Geometry check sheet. Reference: the model listing, model coordinates, mm. Face numbers are marked on the shaded views. A direction names the side the tool comes from. Round coordinates to 2 decimals unless told otherwise and drop trailing zeros. Order: outer loops, then holes, each group sorted by start corner. A loop starts at its lowest first (then second) coordinate and runs counter-clockwise, first axis right, second up. Notation, with made-up numbers: (-34.5, 65.25) - (-29.5, 65.25) arc R10 cw to (-29.5, 74.25) - close; hole circle Ø4 at (17.5, -1). An arc over 180 degrees is marked (long way). Write each question's results on one line, items separated by ' | '.
```python
from build123d import *

# Parameters (mm, degrees)
SKETCH1_R             = 4.765
BOSS_EXTRUDE1_DEPTH   = 9.5
CHAMFER1_SIZE         = 2.54
CHAMFER1_SIZE2        = 7.62
CHAMFER1_PART_2_SIZE  = 2.54
CHAMFER1_PART_2_SIZE2 = 7.62
CHAMFER2_SIZE         = 7.62
CHAMFER2_SIZE2        = 2.54
CUT_EXTRUDE1_DEPTH    = 17
SKETCH3_W             = 9.53
SKETCH3_H             = 9.53
CUT_EXTRUDE2_DEPTH    = 17
SKETCH4_R             = 1.59
CUT_EXTRUDE3_DEPTH    = 17


with BuildPart() as part:
    # Sketch1 → Boss-Extrude1 (new body, symmetric)
    with BuildSketch(Plane(origin=(0, 0, 0), x_dir=(0, 0, -1), z_dir=(1, 0, 0))):
        with BuildLine():
            Line((0, 9.765), (-22.53, 9.765))
            Line((-22.53, 9.765), (-22.53, 4.765))
            Line((-22.53, 4.765), (-9.688074689, -1.223288118))
            ThreePointArc((-9.688074689, -1.223288118), (-5.812387316, -7.84674319), (1.653013564, -9.624072483))
            Line((1.653013564, -9.624072483), (28.575, -5))
            Line((28.575, -5), (28.575, 0))
            Line((28.575, 0), (9.765, 0))
            ThreePointArc((9.765, 0), (6.904897718, 6.904897718), (0, 9.765))
        make_face()
        Circle(SKETCH1_R, mode=Mode.SUBTRACT)
    extrude(amount=BOSS_EXTRUDE1_DEPTH, both=True)

    # Chamfer1
    chamfer1_edges = [part.edges().sort_by_distance(p)[0] for p in [
        (9.5, 7.265, 22.53),
    ]]
    chamfer1_side = [part.faces().sort_by_distance(p)[0] for p in [
        (0, 7.265, 22.53),
    ]]
    chamfer(chamfer1_edges, length=CHAMFER1_SIZE, length2=CHAMFER1_SIZE2, reference=chamfer1_side[0])

    # Chamfer1 part 2
    chamfer1_part_2_edges = [part.edges().sort_by_distance(p)[0] for p in [
        (9.5, -2.5, -28.575),
    ]]
    chamfer1_part_2_side = [part.faces().sort_by_distance(p)[0] for p in [
        (0, -2.5, -28.575),
    ]]
    chamfer(chamfer1_part_2_edges, length=CHAMFER1_PART_2_SIZE, length2=CHAMFER1_PART_2_SIZE2, reference=chamfer1_part_2_side[0])

    # Chamfer2
    chamfer2_edges = [part.edges().sort_by_distance(p)[0] for p in [
        (-9.5, 7.265, 22.53),
        (-9.5, -2.5, -28.575),
    ]]
    chamfer2_side = [part.faces().sort_by_distance(p)[0] for p in [
        (-9.5, 9.217903854, 11.265),
    ]]
    chamfer(chamfer2_edges, length=CHAMFER2_SIZE, length2=CHAMFER2_SIZE2, reference=chamfer2_side[0])

    # Sketch2 → Cut-Extrude1 (cut, symmetric)
    with BuildSketch(Plane(origin=(0, 0, 0), x_dir=(1, 0, 0), z_dir=(0, 1, 0))):
        with BuildLine():
            Line((5.08, 6.35), (5.08, -3.81))
            ThreePointArc((5.08, -3.81), (0, -8.89), (-5.08, -3.81))
            Line((-5.08, -3.81), (-5.08, 6.35))
            ThreePointArc((-5.08, 6.35), (0, 11.43), (5.08, 6.35))
        make_face()
    extrude(amount=CUT_EXTRUDE1_DEPTH, both=True, mode=Mode.SUBTRACT)

    # Sketch3 → Cut-Extrude2 (cut, symmetric)
    with BuildSketch(Plane(origin=(0, 0, 0), x_dir=(1, 0, 0), z_dir=(0, 1, 0))):
        with Locations((0, 23.81)):
            Rectangle(SKETCH3_W, SKETCH3_H)
        with Locations((0, -17.765)):
            Rectangle(SKETCH3_W, SKETCH3_H)
    extrude(amount=CUT_EXTRUDE2_DEPTH, both=True, mode=Mode.SUBTRACT)

    # Sketch4 → Cut-Extrude3 (cut, symmetric)
    with BuildSketch(Plane(origin=(0, 0, 0), x_dir=(0, 0, -1), z_dir=(1, 0, 0))):
        with Locations((26.035, -2.54)):
            Circle(SKETCH4_R)
        with Locations((-19.99, 7.225)):
            Circle(SKETCH4_R)
    extrude(amount=CUT_EXTRUDE3_DEPTH, both=True, mode=Mode.SUBTRACT)


solid = part.part
```
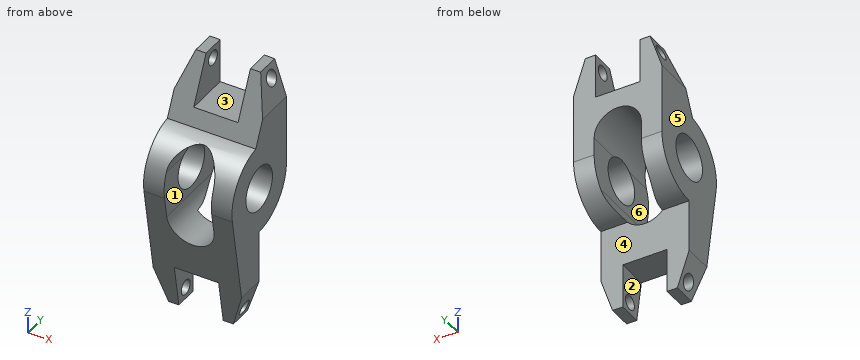
(1) Section check C-C (x = 0). Record the cut outline in (y, z) (3 decimals).
Answers follow:
outline: (-7.945, -11.43) - (-6.637, -19.045) - (0, -19.045) - (0, -11.43) - close; (-4.04, 8.89) - (9.765, 8.89) - (9.765, 13) - (0.321, 13) - (-1.223, 9.688) arc R9.765 ccw to start
(2) Access from +Z, -Z, +X, -X, +Y, -Y to the whole of each face (thin tool, end or side, straight path). Record for the marked faces 1, 2 and 3.
Answers follow:
face 1: +Y, -Y | face 2: -Z, +Y, -Y | face 3: +Z, +Y, -Y
(3) Draft check along X on the marked faces 4, 5 and 6. Enter one of: released by +X, released by -X, zero draft, split by the parting line, or undercut.
Answers follow:
face 4: zero draft | face 5: released by -X | face 6: undercut
(4) Section check A-A (y = 4). Record the cut outline in (x, z) (3 decimals), then the cut area to 3 significant figures.
Answers follow:
outline: (-9.5, -8.908) - (-4.389, -8.908) arc R5.08 cw to (-5.08, -6.35) - (-5.08, -2.589) - (-9.5, -2.589) - close; (-9.5, 2.589) - (-5.08, 2.589) - (-5.08, 3.81) arc R5.08 cw to (5.08, 3.81) - (5.08, 2.589) - (9.5, 2.589) - (9.5, 14.91) - (7.507, 20.889) - (4.765, 20.889) - (4.765, 13) - (-4.765, 13) - (-4.765, 20.889) - (-7.507, 20.889) - (-9.5, 14.91) - close; (4.389, -8.908) - (9.5, -8.908) - (9.5, -2.589) - (5.08, -2.589) - (5.08, -6.35) arc R5.08 cw to start | area: 265 mm²
(5) Material ranges on line 1 (X direction, y = -4.25, z = -5.5); line 2 (Y direction, x = -6.4, z = 19.99) (3 decimals); line 3 (Z direction, x = 4.5, y = -2.25) (3 decimals), recorded low to high.
Answers follow:
line 1: -9.5 to -5.08, 5.08 to 9.5 | line 2: 3.581 to 5.635, 8.815 to 9.765 | line 3: -19.045 to -8.707, 6.167 to 9.502
(6) Section check B-B (x = -6). Record the cut outline in (y, z) (3 decimals).
Answers follow:
outline: (-9.624, -1.653) - (-5, -28.575) - (0, -28.575) - (0, -9.765) arc R9.765 ccw to (9.765, 0) - (9.765, 22.53) - (4.765, 22.53) - (-1.223, 9.688) arc R9.765 ccw to start; hole circle Ø9.53 at (0, 0); hole circle Ø3.18 at (-2.54, -26.035); hole circle Ø3.18 at (7.225, 19.99)
(7) Depth check by flat-ended pin: pin 1 Ø5.5 at (x, y) = (-1, -2.5) entering from -Z (3 decimals); pin 2 Ø5 at (y, z) = (3.5, -12.5) entering from -X; pin 3 Ø5 at (y, z) = (-2.54, -26.035) entering from -X; pin 4 Ø4 at (y, z) = (7.225, 19.99) entering from +X. Enter the tip coordinate at first touch or a pass-through.
Answers follow:
pin 1: z = -19.045 | pin 2: through | pin 3: x = -8.64 | pin 4: x = 8.47
(8) Section check D-D (z = -16.5). Record the cut outline in (x, y), then the cut area to 3 significant figures.
Answers follow:
outline: (-9.5, -7.07) - (9.5, -7.07) - (9.5, 0) - (-9.5, 0) - close | area: 134 mm²
